Geometry check sheet. Reference: the model listing, model coordinates, mm. Round coordinates to 2 decimals unless told otherwise and drop trailing zeros. Loops run counter-clockwise (first coordinate to the right, second up) from the corner with the lowest first, then second, coordinate; pieces in that order, holes last. Notation, with made-up numbers: (4.25, 40) - (8.25, 40) arc R26 ccw to (8.25, 64) - close; hole circle Ø4 at (84.25, 37.5). An arc over 180 degrees is marked (long way). Answer in a Markdown table with one row per item. Add a question column.
```python
from build123d import *

# Parameters (mm, degrees)
SKETCH1_W           = 33.528
SKETCH1_H           = 12.7
BOSS_EXTRUDE1_DEPTH = 2.54
FILLET1_R           = 2.54
SKETCH2_R           = 1.905
SKETCH2_R_2         = 1.27
CUT_EXTRUDE1_DEPTH  = 36.942570637


with BuildPart() as part:
    # Sketch1 → Boss-Extrude1 (new body)
    with BuildSketch(Plane.XY):
        with Locations((-16.764, 6.35)):
            Rectangle(SKETCH1_W, SKETCH1_H)
    extrude(amount=BOSS_EXTRUDE1_DEPTH)

    # Fillet1
    fillet1_edges = [part.edges().sort_by_distance(p)[0] for p in [
        (0, 0, 1.27),
        (-33.528, 0, 1.27),
        (-33.528, 12.7, 1.27),
        (0, 12.7, 1.27),
    ]]
    fillet(fillet1_edges, radius=FILLET1_R)

    # Sketch2 → Cut-Extrude1 (cut, through all)
    with BuildSketch(Plane.XY.offset(2.54)):
        with Locations((-27.178, 6.35)):
            Circle(SKETCH2_R)
        with Locations((-6.858, 6.35)):
            Circle(SKETCH2_R_2)
    extrude(amount=-CUT_EXTRUDE1_DEPTH, mode=Mode.SUBTRACT)


solid = part.part
```
Q1. Scan lines: line 1 (X direction, y = 6.5, z = 1.5); line 2 (X direction, y = 7.25, z = 2.15); line 3 (Y direction, x = -27.5, z = 1.5). Record each from-to range of solid material in increasing order. Write a range as from..to.
Q2. Cross-section at A-A, the plane y = 6.35. Enter the section's corners in (x, z), plus the area to 3 significant figures.
Q3. Release check for a two-part mould opening along Y. For faces 1 (the flat face through (-17, 12.7, 1)), 2 (the flat face through (-33.528, 6, 1)), 3 (the cylindrical face through (-8.127, 6.406, 1.288)) record: +Y half, -Y half, draft (parallel to the pull), parting line (faces both ways), or undercut.
Q4. Cross-section at B-B, the plane z = 1.3. Enter the section's corners in (x, y) (3 decimals), plus the area to 3 significant figures.
Q5. Cross-section at C-C, the plane y = 11.75. Enter the section's corners in (x, z), plus the area to 3 significant figures.
Check sheet entries:
| question | item | result |
|---|---|---|
| 1 | line 1 | -33.53..-29.08, -25.28..-8.12, -5.6..0 |
| 1 | line 2 | -33.53..-28.86, -25.5..-7.75, -5.96..0 |
| 1 | line 3 | 0..4.47, 8.23..12.7 |
| 2 | outline | (-33.53, 0) - (-29.08, 0) - (-29.08, 2.54) - (-33.53, 2.54) - close; (-25.27, 0) - (-8.13, 0) - (-8.13, 2.54) - (-25.27, 2.54) - close; (-5.59, 0) - (0, 0) - (0, 2.54) - (-5.59, 2.54) - close |
| 2 | area | 69.0 mm² |
| 3 | face 1 | +Y half |
| 3 | face 2 | draft |
| 3 | face 3 | undercut |
| 4 | outline | (-33.528, 2.54) arc R2.54 ccw to (-30.988, 0) - (-2.54, 0) arc R2.54 ccw to (0, 2.54) - (0, 10.16) arc R2.54 ccw to (-2.54, 12.7) - (-30.988, 12.7) arc R2.54 ccw to (-33.528, 10.16) - close; hole circle Ø3.81 at (-27.178, 6.35); hole circle Ø2.54 at (-6.858, 6.35) |
| 4 | area | 404 mm² |
| 5 | outline | (-32.97, 0) - (-0.56, 0) - (-0.56, 2.54) - (-32.97, 2.54) - close |
| 5 | area | 82.3 mm² |
